The model under review builds one solid part; all positions refer to its coordinate system, in mm. A direction names the side the tool comes from. Coordinates: 2 decimals unless noted, no trailing zeros. Order: outer loops, then holes, each group sorted by start corner. A loop starts at its lowest first (then second) coordinate and runs counter-clockwise, first axis right, second up. Notation, with made-up numbers: (-2.5, -38) -> (18.5, -38) arc R25 ccw to (18.5, -21) -> close; hole circle Ø2 at (49.25, 1.25). An arc over 180 degrees is marked (long way). Use CSV: the item, a comma, the result in double quotes. Start each with the question number.
```python
from build123d import *

# Parameters (mm, degrees)
F0_W     = 310
F0_H     = 310
F0_W_2   = 250
F0_H_2   = 250
F1_DEPTH = 75
F3_W     = 250
F3_H     = 280
F4_DEPTH = 25
F5_W     = 250
F5_H     = 30
F6_DEPTH = 20
F7_W     = 250
F7_H     = 30
F8_DEPTH = 20


with BuildPart() as f1:
    # F0 (on Top) → F1 (new body, symmetric)
    with BuildSketch(Plane.XY):
        Rectangle(F0_W, F0_H)
        Rectangle(F0_W_2, F0_H_2, mode=Mode.SUBTRACT)
    extrude(amount=F1_DEPTH, both=True)

    # F3 (on offset) → F4 (cut)
    with BuildSketch(Plane.XY.offset(75)):
        Rectangle(F3_W, F3_H)
    extrude(amount=-F4_DEPTH, mode=Mode.SUBTRACT)

    # F5 (on face) → F6 (join)
    with BuildSketch(Plane(origin=(-155, 0, 0), x_dir=(0, -1, 0), z_dir=(-1, 0, 0))):
        Rectangle(F5_W, F5_H)
    extrude(amount=F6_DEPTH)

    # F7 (on face) → F8 (join)
    with BuildSketch(Plane.YZ.offset(155)):
        Rectangle(F7_W, F7_H)
    extrude(amount=F8_DEPTH)


solid = f1.part
```
Q1. Add section B-B, the plane z = 63.5. State the section outline as (x, y) points.
Q2. Draft analysis for pull direction Y (two halves, no side actions). For faces 6 (the flat face through (-2, 125, -12)), 7 (the flat face through (-165, 125, 0)), 8 (the flat face through (-2, 140, 63)), 9 (the flat face through (-165, 2, 15)), state which applies: +Y half, -Y half, draft (parallel to the pull), parting line (faces both ways), or undercut.
Q3. Add section C-C, the plane x = 27. State the section outline as (y, z) points.
Q4. To check wall thickness, follow probe 1 along Y at (x, z) = (-116.5, 22); probe 2 along X at (y, z) = (-89.5, -6). State the ranges of each line that lie inside material, in increasing order.
Q5. Clearance check with flat-ended pins moving along their axes: pin 1 Ø10 at (x, y) = (167.5, 39) entering from +Z; pin 2 Ø6 at (x, y) = (169, 31.5) entering from -Z; pin 3 Ø10 at (x, z) = (169, 5) entering from +Y. State where each tip first meets the part, or that it passes through.
Q6. Add section D-D, the plane z = 29. State the section outline as (x, y) points, then the cut area to 3 significant figures.
Q7. Add section A-A, the plane y = 64.5. State the section outline as (x, z) points.
Q8. For faces 1 (the flat face through (-165, 2, -15)), 2 (the flat face through (165, -125, 0)), 3 (the flat face through (165, -2, 15)), 4 (the flat face through (-2, -132, 50)), 5 (the flat face through (-165, -125, 0)), list the 3-axis set-ups (+Z, -Z, +X, -X, +Y, -Y) from which the entire face can be reached by the end or side of a thin tool; tool diameter is ignored.
Answer block:
1,outline,"(-155, -155) -> (155, -155) -> (155, 155) -> (-155, 155) -> close; hole (-125, -140) -> (125, -140) -> (125, 140) -> (-125, 140) -> close"
2,face 6,"undercut"
2,face 7,"+Y half"
2,face 8,"undercut"
2,face 9,"draft"
3,outline,"(-155, -75) -> (-125, -75) -> (-125, 50) -> (-140, 50) -> (-140, 75) -> (-155, 75) -> close; (125, -75) -> (155, -75) -> (155, 75) -> (140, 75) -> (140, 50) -> (125, 50) -> close"
4,probe 1,"y = -155 to -125, 125 to 155"
4,probe 2,"x = -175 to -125, 125 to 175"
5,pin 1,"stops at z = 15"
5,pin 2,"stops at z = -15"
5,pin 3,"stops at y = 125"
6,outline,"(-155, -155) -> (155, -155) -> (155, 155) -> (-155, 155) -> close; hole (-125, -125) -> (125, -125) -> (125, 125) -> (-125, 125) -> close"
6,area,"33,600 mm²"
7,outline,"(-175, -15) -> (-155, -15) -> (-155, -75) -> (-125, -75) -> (-125, 75) -> (-155, 75) -> (-155, 15) -> (-175, 15) -> close; (125, -75) -> (155, -75) -> (155, -15) -> (175, -15) -> (175, 15) -> (155, 15) -> (155, 75) -> (125, 75) -> close"
8,face 1,"-Z, -X, +Y, -Y"
8,face 2,"+Z, -Z, +X, -Y"
8,face 3,"+Z, +X, +Y, -Y"
8,face 4,"+Z"
8,face 5,"+Z, -Z, -X, -Y"
